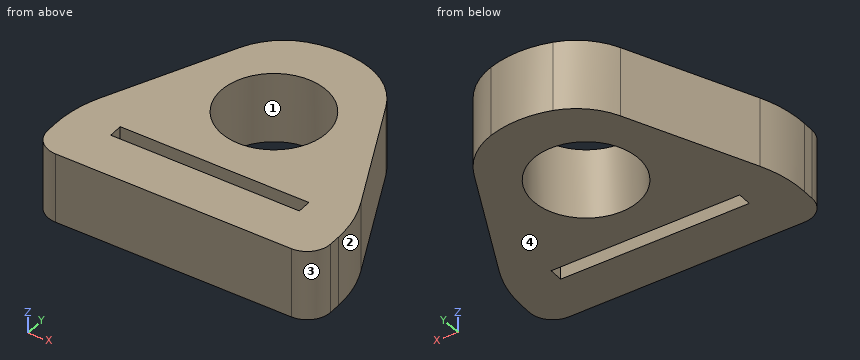
Autodesk Fusion 360 part; units mm, degrees
sketch "Skizze1" plane through (0, 0, 0) normal (0, 0, 1) x (1, 0, 0)
  line L0 (0, 0) -> (8, 0)
  line L1 (8, 0) -> (8, 0.6)
  line L2 (8, 0.6) -> (0, 0.6)
  line L3 (0, 0.6) -> (0, 0)
  circle A0 centre (4, 4.35) radius 2.25
  line L4 (-1, -2) -> (9, -2)
  line L5 (10, -1) -> (10, -0.5092)
  line L6 (-2, -1) -> (-2, -0.5092)
  line L7 (-1.5309, 1.6052) -> (0.8971, 6.808)
  line L8 (9.5309, 1.6052) -> (7.1029, 6.808)
  arc A1 (5.3069, 8.3939) -> (2.6931, 8.3939) centre (4, 4.3499) ccw
  arc A2 (-1.5309, 1.6052) -> (-2, -0.5092) centre (3, -0.5092) ccw
  arc A3 (10, -0.5092) -> (9.5309, 1.6052) centre (5, -0.5092) ccw
  arc A4 (-2, -1) -> (-1, -2) centre (-1, -1) ccw
  arc A5 (9, -2) -> (10, -1) centre (9, -1) ccw
  arc A6 (7.1029, 6.808) -> (5.3069, 8.3939) centre (4.3844, 5.5393) ccw
  arc A7 (2.6931, 8.3939) -> (0.8971, 6.808) centre (3.6156, 5.5393) ccw
  dimension "d1" = 8
  dimension "d2" = 0.6
  dimension "d3" = 4.5
  dimension "d14" = 5
  dimension "d15" = 5
  dimension "d16" = 1
  dimension "d17" = 1
  dimension "d18" = 3
  dimension "d19" = 3
extrude "Extrusion1" add sketch "Skizze1" along normal blind 2
extrude "Extrusion2" add 1 faces at (5.3333, -1.3333, 2) along direction (0, 0, 1) blind 1
Source: CAD feature listing. Evaluate the final solid. Frame: model axes, mm. Face numbers are marked on the shaded views. Give positions to 0.01 mm unless a question says otherwise; leave off trailing zeros. Loops run counter-clockwise (first coordinate to the right, second up) from the corner with the lowest first, then second, coordinate; pieces in that order, holes last. Notation, with made-up numbers: (79.25, 68.25) -> (107.25, 68.25) arc R15 cw to (107.25, 75.25) -> close; hole circle Ø8 at (-2.5, 88). An arc over 180 degrees is marked (long way). Use a Markdown table: item, result. Add a question column.
(1) Section query D-D (x = 0.75). Output: boundary loops of the cut face in (y, z), then the cut area to 3 significant figures.
(2) First-contact query: pin 1 Ø1 at (x, y) = (4, 5.5) entering from +Z; pin 2 Ø1 at (y, z) = (3, 1) entering from +X; pin 3 Ø1 at (y, z) = (3.5, 2.5) entering from +X. Flat tips, straight axial feed; report the tip coordinate or a pass-through.
(3) Ray query, line 1 (Y direction, x = 4, z = 1.15); line 2 (Y direction, x = 5, z = 0.2); line 3 (X direction, y = 6.25, z = 0.4). Return the intervals inside material, ascending.
(4) Section query B-B (x = 4). Output: boundary loops of the cut face in (y, z).
(5) Section query C-C (y = 3.5). Output: boundary loops of the cut face in (x, z), then the cut area to 3 significant figures.
(6) Section query A-A (z = 2.1). Output: boundary loops of the cut face in (x, y).
(7) Pull-direction query (Y, two-part tool) for the marked faces 1, 2, 3 and 4; classes: +Y half, -Y half, draft (parallel to the pull), parting line (faces both ways), or undercut.
Checked values:
| question | item | result |
|---|---|---|
| 1 | outline | (-2, 0) -> (0, 0) -> (0, 3) -> (-2, 3) -> close; (0.6, 0) -> (6.49, 0) -> (6.49, 3) -> (0.6, 3) -> close |
| 1 | area | 23.7 mm^2 |
| 2 | pin 1 | through |
| 2 | pin 2 | x = 9.11 |
| 2 | pin 3 | x = 8.88 |
| 3 | line 1 | -2 to 0, 0.6 to 2.1, 6.6 to 8.6 |
| 3 | line 2 | -2 to 0, 0.6 to 2.33, 6.37 to 8.48 |
| 3 | line 3 | 0.64 to 2.79, 5.21 to 7.36 |
| 4 | outline | (-2, 0) -> (0, 0) -> (0, 3) -> (-2, 3) -> close; (0.6, 0) -> (2.1, 0) -> (2.1, 3) -> (0.6, 3) -> close; (6.6, 0) -> (8.6, 0) -> (8.6, 3) -> (6.6, 3) -> close |
| 5 | outline | (-0.65, 0) -> (1.92, 0) -> (1.92, 3) -> (-0.65, 3) -> close; (6.08, 0) -> (8.65, 0) -> (8.65, 3) -> (6.08, 3) -> close |
| 5 | area | 15.4 mm^2 |
| 6 | outline | (-2, -1) arc R1 ccw to (-1, -2) -> (9, -2) arc R1 ccw to (10, -1) -> (10, -0.51) arc R5 ccw to (9.53, 1.61) -> (7.1, 6.81) arc R3 ccw to (5.31, 8.39) arc R4.25 ccw to (2.69, 8.39) arc R3 ccw to (0.9, 6.81) -> (-1.53, 1.61) arc R5 ccw to (-2, -0.51) -> close; hole (0, 0) -> (8, 0) -> (8, 0.6) -> (0, 0.6) -> close; hole circle Ø4.5 at (4, 4.35) |
| 7 | face 1 | undercut |
| 7 | face 2 | +Y half |
| 7 | face 3 | -Y half |
| 7 | face 4 | draft |
